from build123d import *

# Parameters (mm, degrees)
SKETCH_R        = 60
PAD_DEPTH       = 18
SKETCH001_R     = 2.1
POCKET_DEPTH    = 15.5
SKETCH002_W     = 7.2
SKETCH002_H     = 3.6
POCKET001_DEPTH = 56.1
CHAMFER_1_SIZE2 = 3.59
CHAMFER_1_SIZE  = 2.07
CHAMFER_2_SIZE2 = 3.59
CHAMFER_2_SIZE  = 2.07
CHAMFER_3_SIZE2 = 3.59
CHAMFER_3_SIZE  = 2.07
CHAMFER_4_SIZE2 = 3.59
CHAMFER_4_SIZE  = 2.07
SKETCH003_R     = 4
SKETCH003_R_2   = 10
POCKET002_DEPTH = 2.501
POCKET003_DEPTH = 60
SKETCH005_R     = 2.1
PAD001_DEPTH    = 0.2
SKETCH006_W     = 97
SKETCH006_H     = 10
POCKET004_DEPTH = 10.99


with BuildPart() as part:
    # Sketch → Pad (new body)
    with BuildSketch(Plane.XY):
        Circle(SKETCH_R)
    extrude(amount=PAD_DEPTH)

    # Sketch001 (on Face3 of Pad) → Pocket (cut)
    with BuildSketch(Plane.XY.offset(18)):
        with Locations((-52, 0)):
            Circle(SKETCH001_R)
        with Locations((52, 0)):
            Circle(SKETCH001_R)
        with BuildLine():
            ThreePointArc((-57.784081, -5), (0, -58), (57.784081, -5))
            Line((57.784081, -5), (52, -5))
            ThreePointArc((52, 5), (47, 0), (52, -5))
            Line((52, 5), (57.784081, 5))
            ThreePointArc((57.784081, 5), (0, 58), (-57.784081, 5))
            Line((-57.784081, 5), (-52, 5))
            ThreePointArc((-52, -5), (-47, 0), (-52, 5))
            Line((-52, -5), (-57.784081, -5))
        make_face()
    extrude(amount=-POCKET_DEPTH, mode=Mode.SUBTRACT)

    # Sketch002 → Pocket001 (cut, symmetric)
    with BuildSketch(Plane.YZ):
        with Locations((0, 8.8)):
            Rectangle(SKETCH002_W, SKETCH002_H)
    extrude(amount=POCKET001_DEPTH, both=True, mode=Mode.SUBTRACT)

    # Chamfer 1
    chamfer_1_edges = [part.edges().sort_by_distance(p)[0] for p in [
        (-56.1, -3.6, 8.8),
    ]]
    chamfer_1_side = part.faces().sort_by_distance((-52.315065, -3.6, 8.8))[0]
    chamfer(chamfer_1_edges, length=CHAMFER_1_SIZE, length2=CHAMFER_1_SIZE2, reference=chamfer_1_side)

    # Chamfer 2
    chamfer_2_edges = [part.edges().sort_by_distance(p)[0] for p in [
        (-56.1, 3.6, 8.8),
    ]]
    chamfer_2_side = part.faces().sort_by_distance((-52.315065, 3.6, 8.8))[0]
    chamfer(chamfer_2_edges, length=CHAMFER_2_SIZE, length2=CHAMFER_2_SIZE2, reference=chamfer_2_side)

    # Chamfer 3
    chamfer_3_edges = [part.edges().sort_by_distance(p)[0] for p in [
        (56.1, 3.6, 8.8),
    ]]
    chamfer_3_side = part.faces().sort_by_distance((52.315065, 3.6, 8.8))[0]
    chamfer(chamfer_3_edges, length=CHAMFER_3_SIZE, length2=CHAMFER_3_SIZE2, reference=chamfer_3_side)

    # Chamfer 4
    chamfer_4_edges = [part.edges().sort_by_distance(p)[0] for p in [
        (56.1, -3.6, 8.8),
    ]]
    chamfer_4_side = part.faces().sort_by_distance((52.315065, -3.6, 8.8))[0]
    chamfer(chamfer_4_edges, length=CHAMFER_4_SIZE, length2=CHAMFER_4_SIZE2, reference=chamfer_4_side)

    # Sketch003 (on Face12 of Chamfer) → Pocket002 (cut, through all)
    with BuildSketch(Plane.XY.offset(2.5)):
        with Locations((-33.587572, 33.587572)):
            Circle(SKETCH003_R)
        with Locations((33.587572, -33.587572)):
            Circle(SKETCH003_R)
        with Locations((33.587572, 33.587572)):
            Circle(SKETCH003_R)
        with Locations((-33.587572, -33.587572)):
            Circle(SKETCH003_R)
        with Locations((0, 33)):
            Circle(SKETCH003_R_2)
        Polygon((-21.5, 11.5), (21.5, 11.5), (21.5, -33.5), (11, -33.5), (11, -45.5), (-11, -45.5), (-11, -33.5), (-21.5, -33.5), align=None)
    extrude(amount=-POCKET002_DEPTH, mode=Mode.SUBTRACT)

    # Sketch004 (on Face10 of Pocket002) → Pocket003 (cut)
    with BuildSketch(Plane.XZ.offset(5)):
        with BuildLine():
            ThreePointArc((-5, 12), (-8, 9), (-5, 6))
            Line((-5, 6), (5, 6))
            ThreePointArc((5, 6), (8, 9), (5, 12))
            Line((-5, 12), (5, 12))
        make_face()
    extrude(amount=POCKET003_DEPTH, mode=Mode.SUBTRACT)

    # Sketch005 (on Face1 of Pocket003) → Pad001 (join)
    with BuildSketch(Plane(origin=(0, 0, 10.6), x_dir=(1, 0, 0), z_dir=(0, 0, -1))):
        with Locations((-52, 0)):
            Circle(SKETCH005_R)
        with Locations((52, 0)):
            Circle(SKETCH005_R)
    extrude(amount=-PAD001_DEPTH)

    # Sketch006 (on Face11 of Pad001) → Pocket004 (cut)
    with BuildSketch(Plane.XY.offset(18)):
        Rectangle(SKETCH006_W, SKETCH006_H)
    extrude(amount=-POCKET004_DEPTH, mode=Mode.SUBTRACT)


solid = part.part
The listing builds one solid part. Answer for the finished solid, in the listing's coordinates (mm). A direction names the side the tool comes from. Give positions to 0.01 mm unless a question says otherwise; leave off trailing zeros. Write each loop counter-clockwise with the first axis right and the second up, starting at its lowest first coordinate (ties: lowest second). Pieces come first, ordered by that corner, then holes. Notation, with made-up numbers: (84.5, -5.5) -> (115.5, -5.5) arc R17 cw to (115.5, 2.5) -> close; hole circle Ø7 at (5.5, 17.5). An arc over 180 degrees is marked (long way). Use a Markdown table: item, result.
(1) Section C-C, the plane x = -16 is taken. Determine the outline of the cut face in (y, z).
Return value:
| item | result |
|---|---|
| outline | (-57.83, 0) -> (-33.5, 0) -> (-33.5, 2.5) -> (-55.75, 2.5) -> (-55.75, 18) -> (-57.83, 18) -> close; (11.5, 0) -> (57.83, 0) -> (57.83, 18) -> (55.75, 18) -> (55.75, 2.5) -> (11.5, 2.5) -> close |
(2) Section A-A, the plane x = 0 is taken. Determine the outline of the cut face in (y, z), then the cut area to 4 significant figures.
Return value:
| item | result |
|---|---|
| outline | (-60, 0) -> (-45.5, 0) -> (-45.5, 2.5) -> (-58, 2.5) -> (-58, 6) -> (-60, 6) -> close; (-60, 12) -> (-58, 12) -> (-58, 18) -> (-60, 18) -> close; (11.5, 0) -> (23, 0) -> (23, 2.5) -> (11.5, 2.5) -> close; (43, 0) -> (60, 0) -> (60, 18) -> (58, 18) -> (58, 2.5) -> (43, 2.5) -> close |
| area | 157.5 mm2 |
(3) Flat-ended cylindrical pins translate along their axes: P1, Ø6, axis at x = -42.5, z = 3, coming from the -Y side; P2, Ø10, axis at x = 16.5, z = 8.5, coming from the -Y side; P3, Ø8, axis at x = 11.5, z = 2.5, coming from the -Y side. Find the tip coordinate at first contact, or state that the pin passes through.
Return value:
| item | result |
|---|---|
| P1 | y = -45.16 |
| P2 | y = -58.89 |
| P3 | y = -59.53 |
(4) Determine the mould class of faces 5 (the flat face through (55.08, -1.78, 8.77)), 6 (the flat face through (-1, 14, 0)) for opening direction X: released by +X, released by -X, zero draft, split by the parting line, or undercut.
Return value:
| item | result |
|---|---|
| face 5 | undercut |
| face 6 | zero draft |
(5) Find the intervals of material crossed by probe 1 along Y at (x, z) = (0, 1.45); probe 2 along Y at (x, z) = (-52, 16); probe 3 along Z at (x, y) = (19.5, 46), in increasing order. Write a range as from..to.
Return value:
| item | result |
|---|---|
| probe 1 | -60..-45.5, 11.5..23, 43..60 |
| probe 2 | -29.93..-25.69, -5..-2.1, 2.1..5, 25.69..29.93 |
| probe 3 | 0..2.5 |
(6) For faces 1 (the cylindrical face through (-8, -59, 9)), 2 (the flat face through (-48.5, 0, 14)), 3 (the cylindrical face through (-31.74, 30.04, 1.27)), 4 (the flat face through (49.6, -0.1, 7)), determine the directions among +Z, -Z, +X, -X, +Y, -Y from which every point of the face is accessible in a straight line to the end or side of a thin tool.
Return value:
| item | result |
|---|---|
| face 1 | -Y |
| face 2 | +Z |
| face 3 | +Z, -Z |
| face 4 | none |
